Here's how the part is built. I have some questions about the finished solid (model axes, mm). Face numbers are marked on the shaded views. A direction names the side the tool comes from. Coordinates: 2 decimals unless noted, no trailing zeros. Write each loop counter-clockwise with the first axis right and the second up, starting at its lowest first coordinate (ties: lowest second). Pieces come first, ordered by that corner, then holes.
(1) Thinking about a two-plate mould opening in Z: for the marked faces 1, 2 and 3, which applies, released by +Z, released by -Z, zero draft, split by the parting line, or undercut?
(2) Please list where these lines run through material, in increasing order: probe 1 along Z at (x, y) = (0, -109.5); probe 2 along Y at (x, z) = (88, 163); probe 3 along Z at (x, y) = (77, -19).
(3) Imagine slicing it at B-B, the plane x = 62.5. List the corners of the cut face in (y, z) for me (1 decimal).
(4) Imagine slicing it at C-C, the plane x = -89.5. List the corners of the cut face in (y, z) for me (1 decimal), plus the area to 3 significant figures.
(5) For pin 1 Ø3 at (x, z) = (125, 61) entering from -Y; pin 2 Ø12.5 at (x, z) = (-34.925, -34.925) entering from +Y; pin 3 Ø12 at (y, z) = (-89.5, -88.5) entering from -X, each with a flat end and sliding along its axis, tell me the tip position at first contact or that it passes through.
(6) Imagine slicing it at D-D, the plane z = 158. List the corners of the cut face in (x, y) for me, plus the area to 3 significant figures.
(7) Imagine slicing it at A-A, the plane y = -46. List the corners of the cut face in (x, z) for me.
(8) Which directions (+Z, -Z, +X, -X, +Y, -Y) give clear straight access to the entire face, cutting with the end or side of a thin tool? Please do the marked faces 4, 5 and 6.
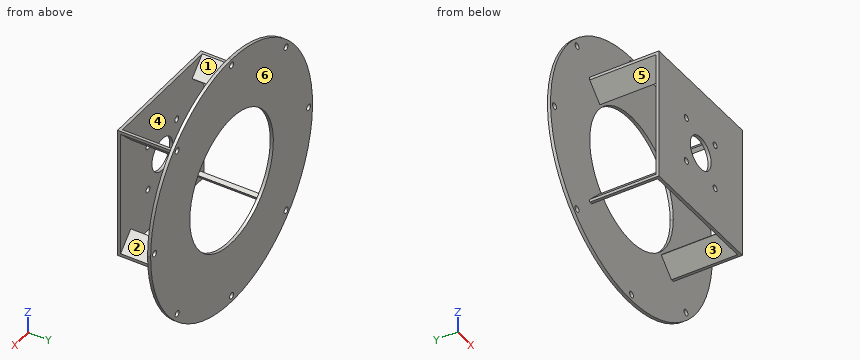
```python
from build123d import *

# Parameters (mm, degrees)
F0_R     = 4.7625
F1_DEPTH = 4.7625
F3_DEPTH = 101.6
F4_W     = 203.2
F4_H     = 203.2
F4_R     = 4.7625
F4_R_2   = 25.4
F5_DEPTH = 4.7625


with BuildPart() as f1:
    # F0 (on Front) → F1 (new body)
    with BuildSketch(Plane.XZ):
        with BuildLine():
            ThreePointArc((196.85, 0), (139.19397, 139.19397), (0, 196.85))
            ThreePointArc((0, 196.85), (-139.19397, -139.19397), (196.85, 0))
        make_face()
        with Locations((-132.458778, -132.458778)):
            Circle(F0_R, mode=Mode.SUBTRACT)
        with Locations((0, -187.325)):
            Circle(F0_R, mode=Mode.SUBTRACT)
        with Locations((132.458778, -132.458778)):
            Circle(F0_R, mode=Mode.SUBTRACT)
        with Locations((-187.325, 0)):
            Circle(F0_R, mode=Mode.SUBTRACT)
        with Locations((-132.458778, 132.458778)):
            Circle(F0_R, mode=Mode.SUBTRACT)
        with BuildLine():
            ThreePointArc((177.8, 0), (-125.723586, -125.723586), (0, 177.8))
            ThreePointArc((0, 177.8), (125.723586, 125.723586), (177.8, 0))
        make_face(mode=Mode.SUBTRACT)
        with Locations((187.325, 0)):
            Circle(F0_R, mode=Mode.SUBTRACT)
        with BuildLine():
            ThreePointArc((4.7625, 187.325), (3.367596, 183.957404), (0, 182.5625))
            ThreePointArc((0, 182.5625), (-4.7625, 187.325), (0, 192.0875))
            ThreePointArc((0, 192.0875), (3.367596, 190.692596), (4.7625, 187.325))
        make_face(mode=Mode.SUBTRACT)
        with Locations((132.458778, 132.458778)):
            Circle(F0_R, mode=Mode.SUBTRACT)
        with BuildLine():
            ThreePointArc((177.8, 0), (125.723586, 125.723586), (0, 177.8))
            ThreePointArc((0, 177.8), (-125.723586, -125.723586), (177.8, 0))
        make_face()
        with BuildLine():
            ThreePointArc((0, 101.6), (71.842049, 71.842049), (101.6, 0))
            ThreePointArc((101.6, 0), (-71.842049, -71.842049), (0, 101.6))
        make_face(mode=Mode.SUBTRACT)
    extrude(amount=F1_DEPTH)

    # F2 (on face) → F3 (join)
    with BuildSketch(Plane.XZ.offset(4.7625)):
        Polygon((-72.414168, 76.904296), (-97.109872, 101.6), (-101.6, 101.6), (-101.6, 97.109872), (-76.904296, 72.414168), (-74.659232, 74.659232), align=None)
        Polygon((76.904296, 72.414168), (101.6, 97.109872), (101.6, 101.6), (97.109872, 101.6), (72.414168, 76.904296), (74.659232, 74.659232), align=None)
        Polygon((101.6, -101.6), (101.6, -97.109872), (76.904296, -72.414168), (74.659232, -74.659232), (72.414168, -76.904296), (97.109872, -101.6), align=None)
        Polygon((-101.6, -101.6), (-97.109872, -101.6), (-72.414168, -76.904296), (-74.659232, -74.659232), (-76.904296, -72.414168), (-101.6, -97.109872), align=None)
    extrude(amount=F3_DEPTH)

    # F4 (on face) → F5 (join)
    with BuildSketch(Plane.XZ.offset(106.3625)):
        Rectangle(F4_W, F4_H)
        with Locations((-34.925, -34.925)):
            Circle(F4_R, mode=Mode.SUBTRACT)
        Circle(F4_R_2, mode=Mode.SUBTRACT)
        with Locations((34.925, -34.925)):
            Circle(F4_R, mode=Mode.SUBTRACT)
        with Locations((-34.925, 34.925)):
            Circle(F4_R, mode=Mode.SUBTRACT)
        with BuildLine():
            ThreePointArc((39.6875, 34.925), (38.292596, 31.557404), (34.925, 30.1625))
            ThreePointArc((34.925, 30.1625), (31.557404, 38.292596), (39.6875, 34.925))
        make_face(mode=Mode.SUBTRACT)
        Polygon((-97.109872, 101.6), (-101.6, 101.6), (-101.6, -101.6), (101.6, -101.6), (101.6, 101.6), align=None)
        with Locations((-34.925, -34.925)):
            Circle(F4_R, mode=Mode.SUBTRACT)
        Circle(F4_R_2, mode=Mode.SUBTRACT)
        with Locations((34.925, -34.925)):
            Circle(F4_R, mode=Mode.SUBTRACT)
        with Locations((-34.925, 34.925)):
            Circle(F4_R, mode=Mode.SUBTRACT)
        with BuildLine():
            ThreePointArc((39.6875, 34.925), (38.292596, 31.557404), (34.925, 30.1625))
            ThreePointArc((34.925, 30.1625), (31.557404, 38.292596), (39.6875, 34.925))
        make_face(mode=Mode.SUBTRACT)
    extrude(amount=F5_DEPTH)


solid = f1.part
```
Recorded:
1. face 1: released by +Z
1. face 2: undercut
1. face 3: released by -Z
2. probe 1: z = -101.6 to -25.4, 25.4 to 101.6
2. probe 2: y = -4.76 to 0
2. probe 3: z = -81.49 to -72.51, 72.51 to 81.49
3. outline: (-111.1, -101.6) - (-106.4, -101.6) - (-106.4, 101.6) - (-111.1, 101.6) - close; (-4.8, -186.7) - (0, -186.7) - (0, -80.1) - (-4.8, -80.1) - close; (-4.8, 80.1) - (0, 80.1) - (0, 186.7) - (-4.8, 186.7) - close
4. outline: (-111.1, -101.6) - (-106.4, -101.6) - (-106.4, -94) - (-4.8, -94) - (-4.8, -175.3) - (0, -175.3) - (0, -48.1) - (-4.8, -48.1) - (-4.8, -85) - (-106.4, -85) - (-106.4, 85) - (-4.8, 85) - (-4.8, 48.1) - (0, 48.1) - (0, 175.3) - (-4.8, 175.3) - (-4.8, 94) - (-106.4, 94) - (-106.4, 101.6) - (-111.1, 101.6) - close
4. area: 4,000 mm2
5. pin 1: stops at y = -4.76
5. pin 2: stops at y = -106.36
5. pin 3: stops at x = -98.99
6. outline: (-117.41, -4.76) - (117.41, -4.76) - (117.41, 0) - (-117.41, 0) - close
6. area: 1,120 mm2
7. outline: (-101.6, -101.6) - (-97.11, -101.6) - (-72.41, -76.9) - (-76.9, -72.41) - (-101.6, -97.11) - close; (-101.6, 97.11) - (-76.9, 72.41) - (-72.41, 76.9) - (-97.11, 101.6) - (-101.6, 101.6) - close; (72.41, -76.9) - (97.11, -101.6) - (101.6, -101.6) - (101.6, -97.11) - (76.9, -72.41) - close; (72.41, 76.9) - (76.9, 72.41) - (101.6, 97.11) - (101.6, 101.6) - (97.11, 101.6) - close
8. face 4: none
8. face 5: -X
8. face 6: +Z, -Z, +X, -X, +Y
